Model file for the job. Use its own axes, mm. A direction names the side the tool comes from. Coordinates: 2 decimals unless noted, no trailing zeros. Write each loop counter-clockwise with the first axis right and the second up, starting at its lowest first coordinate (ties: lowest second). Pieces come first, ordered by that corner, then holes.
Q1. Which spindle directions (+Z, -Z, +X, -X, +Y, -Y) get a long thin tool onto all of the face, cutting with end or side? Do faces 1 (the flat face through (10.1, 5, 32)), 2 (the cylindrical face through (0.358, 12.06, 25.273)), 3 (the flat face through (15, 4, 22)), 4 (the flat face through (0, 14.1, 37)). Say none if no direction does.
Q2. Drill centre lines: probe 1 along Z at (x, y) = (0, 13); probe 2 along Z at (x, y) = (9.5, 5.25); probe 3 along X at (y, z) = (1.25, 48). Where is each one in solid material? Low to high.
Q3. Band-saw the part on D-D, the plane y = 12.25. Write the cut outline in (x, z).
Q4. Band-saw the part on C-C, the plane y = 8. Write the cut outline in (x, z) (3 decimals).
Q5. Pin check, flat tips, straight feed: P1, Ø3, axis at y = 12, z = 32, coming from the -X side; P2, Ø12, axis at x = -13, z = 26.5, coming from the +Y side; P3, Ø9, axis at x = 0, z = 28, coming from the -Y side. Stop position of each tip, or through.
Q6. Band-saw the part on A-A, the plane x = 0. Write the cut outline in (y, z) (3 decimals), plus the area to 3 significant figures.
Q7. Band-saw the part on B-B, the plane z = 43. Write the cut outline in (x, y) (3 decimals), plus the area to 3 significant figures.
Q8. Pull direction Z, two halves, no side cores. Call faces 5 (the flat face through (14.1, 5, 37)), 6 (the flat face through (8, 9, 22)), 7 (the flat face through (0, 11, 12)): released by +Z, released by -Z, zero draft, split by the parting line, or undercut.
from build123d import *

# Parameters (mm, degrees)
SKETCH_1_R                     = 17
EXTRUDE_1_DEPTH                = 2
SKETCH_2_R                     = 17
SKETCH_2_R_2                   = 15
EXTRUDE_2_DEPTH                = 10
SKETCH_3_R                     = 5
CUT_EXTRUDE_1_DEPTH            = 27.038433133
SKETCH_4_R                     = 17
EXTRUDE_3_DEPTH                = 10
SKETCH_5_W                     = 20.2
SKETCH_5_H                     = 20.2
EXTRUDE_4_DEPTH                = 30
HOLE_WIZARD_M5_2_D             = 5.5
HOLE_WIZARD_M5_2_CSINK_D       = 5.55
HOLE_WIZARD_M5_2_CSINK_ANGLE   = 90
HOLE_WIZARD_M2_5_2_D           = 2.9
HOLE_WIZARD_M2_5_2_CSINK_D     = 2.95
HOLE_WIZARD_M2_5_2_CSINK_ANGLE = 90
SKETCH1_W                      = 65
SKETCH1_H                      = 40
CUT_EXTRUDE2_DEPTH             = 58.28874235


with BuildPart() as part:
    # 草图1 → 凸台-拉伸1 (new body)
    with BuildSketch(Plane.XY):
        Circle(SKETCH_1_R)
    extrude(amount=EXTRUDE_1_DEPTH)

    # 草图2 → 凸台-拉伸2 (add)
    with BuildSketch(Plane.XY.offset(2)):
        Circle(SKETCH_2_R)
        Circle(SKETCH_2_R_2, mode=Mode.SUBTRACT)
    extrude(amount=EXTRUDE_2_DEPTH)

    # 草图3 → 切除-拉伸1 (cut, through all)
    with BuildSketch(Plane.XY.offset(2)):
        Circle(SKETCH_3_R)
    extrude(amount=-CUT_EXTRUDE_1_DEPTH, mode=Mode.SUBTRACT)

    # 草图4 → 凸台-拉伸3 (add)
    with BuildSketch(Plane.XY.offset(12)):
        Circle(SKETCH_4_R)
        Polygon((-4.443145751, 10.1), (4.443145751, 10.1), (10.1, 4.443145751), (10.1, -4.443145751), (4.443145751, -10.1), (-4.443145751, -10.1), (-10.1, -4.443145751), (-10.1, 4.443145751), align=None, mode=Mode.SUBTRACT)
    extrude(amount=EXTRUDE_3_DEPTH)

    # 草图5 → 凸台-拉伸4 (add)
    with BuildSketch(Plane.XY.offset(22)):
        with BuildLine():
            Line((9.49684158, 14.1), (-9.49684158, 14.1))
            ThreePointArc((-9.49684158, 14.1), (-12.02081528, 12.02081528), (-14.1, 9.49684158))
            Line((-14.1, 9.49684158), (-14.1, -9.496842588))
            ThreePointArc((-14.1, -9.496842588), (-12.020815678, -12.020815678), (-9.496842588, -14.1))
            Line((-9.496842588, -14.1), (9.49684158, -14.1))
            ThreePointArc((9.49684158, -14.1), (12.02081528, -12.02081528), (14.1, -9.49684158))
            Line((14.1, -9.49684158), (14.1, 9.49684158))
            ThreePointArc((14.1, 9.49684158), (12.02081528, 12.02081528), (9.49684158, 14.1))
        make_face()
        Rectangle(SKETCH_5_W, SKETCH_5_H, mode=Mode.SUBTRACT)
    extrude(amount=EXTRUDE_4_DEPTH)

    # M5 间隙孔2 (through all)
    with Locations(Plane(origin=(0, 14.1, 0), x_dir=(1, 0, 0), z_dir=(0, 1, 0))):
        with Locations((0, -28), (0, -43)):
            CounterSinkHole(HOLE_WIZARD_M5_2_D / 2, HOLE_WIZARD_M5_2_CSINK_D / 2, counter_sink_angle=HOLE_WIZARD_M5_2_CSINK_ANGLE)

    # M2.5 间隙孔2 (through all)
    with Locations(Plane.XY.offset(2)):
        with Locations((0, 8), (5.656854249, 5.656854249), (8, 0), (5.656854249, -5.656854249), (0, -8), (-5.656854249, -5.656854249), (-8, 0), (-5.656854249, 5.656854249)):
            CounterSinkHole(HOLE_WIZARD_M2_5_2_D / 2, HOLE_WIZARD_M2_5_2_CSINK_D / 2, counter_sink_angle=HOLE_WIZARD_M2_5_2_CSINK_ANGLE)

    # Sketch1 → Cut-Extrude2 (cut, through all)
    with BuildSketch(Plane(origin=(0, 0, 0), x_dir=(0, 0, -1), z_dir=(0, 1, 0))):
        with Locations((-30, 0)):
            Rectangle(SKETCH1_W, SKETCH1_H)
    extrude(amount=-CUT_EXTRUDE2_DEPTH, mode=Mode.SUBTRACT)


solid = part.part
Answer sheet:
1. face 1: +Z, -Y
1. face 2: +Y, -Y
1. face 3: +Z, +X, +Y, -Y
1. face 4: +Z, +X, -X, +Y
2. probe 1: z = 0 to 2, 12 to 25.25, 30.75 to 40.25, 45.75 to 52
2. probe 2: z = 0 to 2, 12 to 22
2. probe 3: x = -14.1 to -10.1, 10.1 to 14.1
3. outline: (-11.79, 0) - (11.79, 0) - (11.79, 52) - (-11.79, 52) - close; hole (-8.66, 2) - (8.66, 2) - (8.66, 12) - (-8.66, 12) - close; hole circle Ø5.5 at (0, 28); hole circle Ø5.5 at (0, 43)
4. outline: (-15, 0) - (-1.45, 0) - (-1.45, 1.975) - (-1.475, 2) - (-12.689, 2) - (-12.689, 12) - (-6.543, 12) - (-6.543, 22) - (-10.1, 22) - (-10.1, 52) - (-14.1, 52) - (-14.1, 22) - (-15, 22) - close; (1.45, 0) - (15, 0) - (15, 22) - (14.1, 22) - (14.1, 52) - (10.1, 52) - (10.1, 22) - (6.543, 22) - (6.543, 12) - (12.689, 12) - (12.689, 2) - (1.475, 2) - (1.45, 1.975) - close
5. P1: stops at x = -13.37
5. P2: stops at y = 14.4
5. P3: stops at y = 10.1
6. outline: (5, 0) - (6.55, 0) - (6.55, 1.975) - (6.525, 2) - (5, 2) - close; (9.45, 0) - (17, 0) - (17, 22) - (14.1, 22) - (14.1, 25.225) - (14.075, 25.25) - (10.1, 25.25) - (10.1, 12) - (15, 12) - (15, 2) - (9.475, 2) - (9.45, 1.975) - close; (10.1, 30.75) - (14.075, 30.75) - (14.1, 30.775) - (14.1, 40.225) - (14.075, 40.25) - (10.1, 40.25) - close; (10.1, 45.75) - (14.075, 45.75) - (14.1, 45.775) - (14.1, 52) - (10.1, 52) - close
6. area: 183 mm2
7. outline: (-14.1, 0) - (-10.1, 0) - (-10.1, 10.1) - (-2.75, 10.1) - (-2.75, 14.075) - (-2.775, 14.1) - (-9.497, 14.1) arc R17 ccw to (-14.1, 9.497) - close; (2.75, 10.1) - (10.1, 10.1) - (10.1, 0) - (14.1, 0) - (14.1, 9.497) arc R17 ccw to (9.497, 14.1) - (2.775, 14.1) - (2.75, 14.075) - close
7. area: 153 mm2
8. face 5: zero draft
8. face 6: released by +Z
8. face 7: undercut
